Input: dimensioned drawing with shaded views. Units: mm. Origin: part minimum x, y, z. Round coordinates to 2 decimals unless told otherwise and drop trailing zeros. Order: outer loops, then holes, each group sorted by start corner. A loop starts at its lowest first (then second) coordinate and runs counter-clockwise, first axis right, second up. Notation, with made-up numbers: (-34.75, 47.5) - (-8.75, 47.5) arc R14 cw to (-8.75, 59.5) - close; hole circle Ø1 at (89, 43.5). An arc over 180 degrees is marked (long way). Return JSON: item names as keys, results as strings. Group by question number.
1) Ray query, line 1 (Z direction, x = 25.5, y = 0.8) (1 decimal); line 2 (X direction, y = 0.5, z = 4); line 3 (Z direction, x = 46, y = 0.65). Return the intervals inside material, ascending. Write a range as from..to.
2) Section D-D, the plane z = 16.5. Return loops of the section in (x, y), plus the area to 3 significant figures.
3) Contact query for flat-ended pins moving along their axis: P1, Ø1.2, axis at x = 1.5, y = 0.5, coming from the +Z side; P2, Ø1, axis at y = 1, z = 21, coming from the +X side. Output: stop coordinate, or through.
4) Section A-A, the plane z = 30. Return loops of the section in (x, y) (1 decimal), plus the area to 3 significant figures.
5) Section C-C, the plane x = 18. Return loops of the section in (y, z).
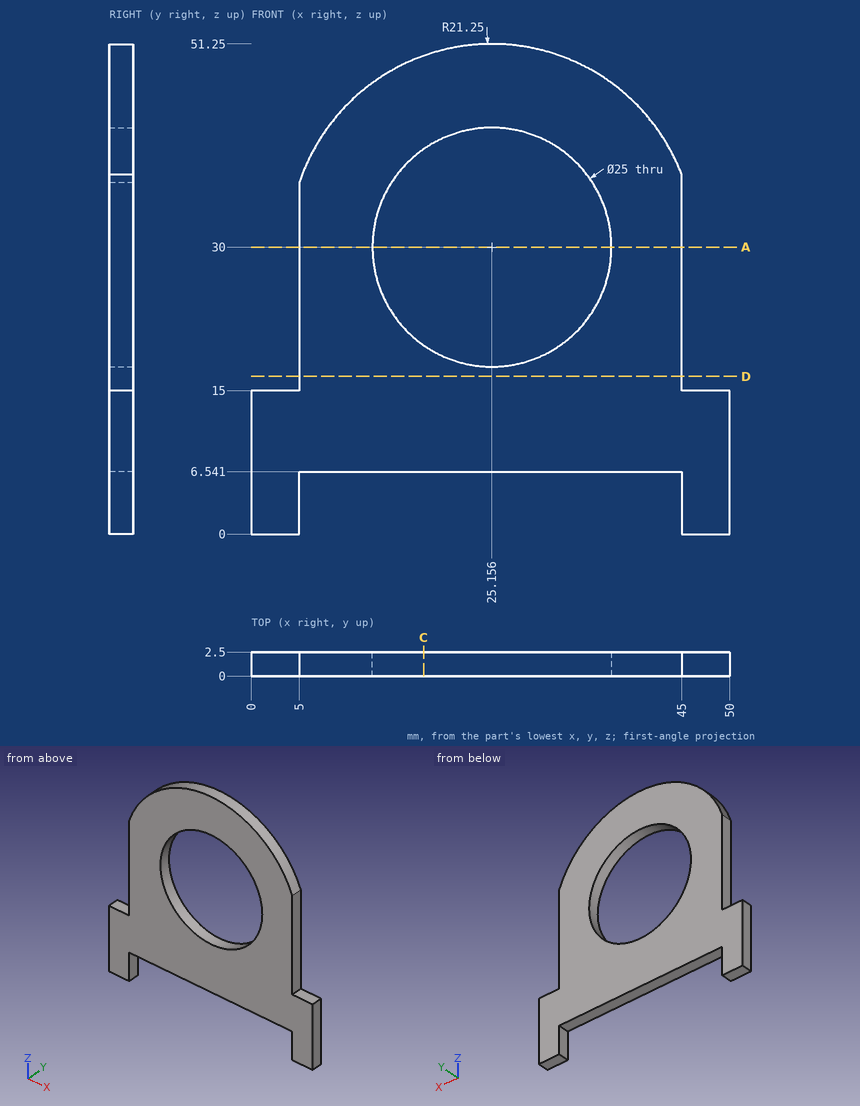
Geometry check:
{
 "1": {"line 1": "6.5..17.5, 42.5..51.2", "line 2": "0..5, 45..50", "line 3": "0..15"},
 "2": {"outline": "(5, 0) - (45, 0) - (45, 2.5) - (5, 2.5) - close", "area": "100 mm2"},
 "3": {"P1": "z = 15", "P2": "x = 45"},
 "4": {"outline": "(5, 0) - (12.7, 0) - (12.7, 2.5) - (5, 2.5) - close; (37.7, 0) - (45, 0) - (45, 2.5) - (37.7, 2.5) - close", "area": "37.5 mm2"},
 "5": {"outline": "(0, 6.54) - (2.5, 6.54) - (2.5, 19.75) - (0, 19.75) - close; (0, 40.25) - (2.5, 40.25) - (2.5, 50.01) - (0, 50.01) - close"}
}
